from build123d import *

# Parameters (mm, degrees)
F0_R     = 4.05
F1_DEPTH = 50
F2_R     = 10.963605
F2_R_2   = 4.05
F3_DEPTH = 100


with BuildPart() as f1:
    # F0 (on Top) → F1 (new body)
    with BuildSketch(Plane.XY):
        with BuildLine():
            Line((14.85866, -53.070427), (16.429462, -41.893589))
            ThreePointArc((16.429462, -41.893589), (9.356026, -44.016642), (2.030598, -44.954162))
            Line((2.030598, -44.954162), (8.011626, -54.525809))
            Line((8.011626, -54.525809), (11.435143, -53.798118))
            Line((11.435143, -53.798118), (14.85866, -53.070427))
        make_face()
        with BuildLine():
            Line((-8.011626, -54.525809), (-2.030598, -44.954162))
            ThreePointArc((-2.030598, -44.954162), (-9.356026, -44.016642), (-16.429462, -41.893589))
            Line((-16.429462, -41.893589), (-14.85866, -53.070427))
            Line((-14.85866, -53.070427), (-11.435143, -53.798118))
            Line((-11.435143, -53.798118), (-8.011626, -54.525809))
        make_face()
        with BuildLine():
            Line((-29.496629, -46.553183), (-20.139548, -40.241752))
            ThreePointArc((-20.139548, -40.241752), (-26.450336, -36.405765), (-32.048718, -31.589234))
            Line((-32.048718, -31.589234), (-35.159748, -42.438686))
            Line((-35.159748, -42.438686), (-32.328189, -44.495935))
            Line((-32.328189, -44.495935), (-29.496629, -46.553183))
        make_face()
        with BuildLine():
            Line((-45.881397, -30.531089), (-34.766188, -28.571178))
            ThreePointArc((-34.766188, -28.571178), (-38.971143, -22.5), (-42.126459, -15.822813))
            Line((-42.126459, -15.822813), (-49.381397, -24.468911))
            Line((-49.381397, -24.468911), (-47.631397, -27.5))
            Line((-47.631397, -27.5), (-45.881397, -30.531089))
        make_face()
        with BuildLine():
            Line((-54.332855, -9.229892), (-43.381438, -11.960387))
            ThreePointArc((-43.381438, -11.960387), (-44.753485, -4.703781), (-44.920154, 2.679516))
            Line((-44.920154, 2.679516), (-55.064554, -2.268239))
            Line((-55.064554, -2.268239), (-54.698704, -5.749065))
            Line((-54.698704, -5.749065), (-54.332855, -9.229892))
        make_face()
        with BuildLine():
            ThreePointArc((-37.916147, 24.23563), (-33.441517, 30.110877), (-28.066181, 35.175126))
            Line((-28.066181, 35.175126), (-38.531008, 39.40319))
            Line((-38.531008, 39.40319), (-40.872965, 36.802183))
            Line((-40.872965, 36.802183), (-43.214923, 34.201176))
            Line((-43.214923, 34.201176), (-37.916147, 24.23563))
        make_face()
        with BuildLine():
            ThreePointArc((-44.495643, 6.718463), (-42.797543, 13.905765), (-39.946745, 20.718532))
            Line((-39.946745, 20.718532), (-51.226549, 20.324632))
            Line((-51.226549, 20.324632), (-52.308108, 16.995935))
            Line((-52.308108, 16.995935), (-53.389668, 13.667237))
            Line((-53.389668, 13.667237), (-44.495643, 6.718463))
        make_face()
        with BuildLine():
            ThreePointArc((-24.780606, 37.562236), (-18.303149, 41.109546), (-11.33272, 43.549621))
            Line((-11.33272, 43.549621), (-19.173106, 51.668578))
            Line((-19.173106, 51.668578), (-22.370515, 50.245))
            Line((-22.370515, 50.245), (-25.567924, 48.821422))
            Line((-25.567924, 48.821422), (-24.780606, 37.562236))
        make_face()
        with BuildLine():
            ThreePointArc((-7.360272, 44.393991), (0, 45), (7.360272, 44.393991))
            Line((7.360272, 44.393991), (3.5, 55))
            Line((3.5, 55), (0, 55))
            Line((0, 55), (-3.5, 55))
            Line((-3.5, 55), (-7.360272, 44.393991))
        make_face()
        with BuildLine():
            ThreePointArc((11.33272, 43.549621), (18.303149, 41.109546), (24.780606, 37.562236))
            Line((24.780606, 37.562236), (25.567924, 48.821422))
            Line((25.567924, 48.821422), (22.370515, 50.245))
            Line((22.370515, 50.245), (19.173106, 51.668578))
            Line((19.173106, 51.668578), (11.33272, 43.549621))
        make_face()
        with BuildLine():
            ThreePointArc((28.066181, 35.175126), (33.441517, 30.110877), (37.916147, 24.23563))
            Line((37.916147, 24.23563), (43.214923, 34.201176))
            Line((43.214923, 34.201176), (40.872965, 36.802183))
            Line((40.872965, 36.802183), (38.531008, 39.40319))
            Line((38.531008, 39.40319), (28.066181, 35.175126))
        make_face()
        with BuildLine():
            ThreePointArc((39.946745, 20.718532), (42.797543, 13.905765), (44.495643, 6.718463))
            Line((44.495643, 6.718463), (53.389668, 13.667237))
            Line((53.389668, 13.667237), (52.308108, 16.995935))
            Line((52.308108, 16.995935), (51.226549, 20.324632))
            Line((51.226549, 20.324632), (39.946745, 20.718532))
        make_face()
        with BuildLine():
            Line((49.381397, -24.468911), (42.126459, -15.822813))
            ThreePointArc((42.126459, -15.822813), (38.971143, -22.5), (34.766188, -28.571178))
            Line((34.766188, -28.571178), (45.881397, -30.531089))
            Line((45.881397, -30.531089), (47.631397, -27.5))
            Line((47.631397, -27.5), (49.381397, -24.468911))
        make_face()
        with BuildLine():
            ThreePointArc((43.381438, -11.960387), (44.593524, -6.034704), (45, 0))
            ThreePointArc((45, 0), (44.980034, 1.340353), (44.920154, 2.679516))
            ThreePointArc((44.920154, 2.679516), (44.753485, 4.703781), (44.495643, 6.718463))
            ThreePointArc((44.495643, 6.718463), (42.797543, 13.905765), (39.946745, 20.718532))
            ThreePointArc((39.946745, 20.718532), (38.971143, 22.5), (37.916147, 24.23563))
            ThreePointArc((37.916147, 24.23563), (33.441517, 30.110877), (28.066181, 35.175126))
            ThreePointArc((28.066181, 35.175126), (26.450336, 36.405765), (24.780606, 37.562236))
            ThreePointArc((24.780606, 37.562236), (18.303149, 41.109546), (11.33272, 43.549621))
            ThreePointArc((11.33272, 43.549621), (9.356026, 44.016642), (7.360272, 44.393991))
            ThreePointArc((7.360272, 44.393991), (0, 45), (-7.360272, 44.393991))
            ThreePointArc((-7.360272, 44.393991), (-9.356026, 44.016642), (-11.33272, 43.549621))
            ThreePointArc((-11.33272, 43.549621), (-18.303149, 41.109546), (-24.780606, 37.562236))
            ThreePointArc((-24.780606, 37.562236), (-26.450336, 36.405765), (-28.066181, 35.175126))
            ThreePointArc((-28.066181, 35.175126), (-33.441517, 30.110877), (-37.916147, 24.23563))
            ThreePointArc((-37.916147, 24.23563), (-38.971143, 22.5), (-39.946745, 20.718532))
            ThreePointArc((-39.946745, 20.718532), (-42.797543, 13.905765), (-44.495643, 6.718463))
            ThreePointArc((-44.495643, 6.718463), (-44.753485, 4.703781), (-44.920154, 2.679516))
            ThreePointArc((-44.920154, 2.679516), (-44.753485, -4.703781), (-43.381438, -11.960387))
            ThreePointArc((-43.381438, -11.960387), (-42.797543, -13.905765), (-42.126459, -15.822813))
            ThreePointArc((-42.126459, -15.822813), (-38.971143, -22.5), (-34.766188, -28.571178))
            ThreePointArc((-34.766188, -28.571178), (-33.441517, -30.110877), (-32.048718, -31.589234))
            ThreePointArc((-32.048718, -31.589234), (-26.450336, -36.405765), (-20.139548, -40.241752))
            ThreePointArc((-20.139548, -40.241752), (-18.303149, -41.109546), (-16.429462, -41.893589))
            ThreePointArc((-16.429462, -41.893589), (-9.356026, -44.016642), (-2.030598, -44.954162))
            ThreePointArc((-2.030598, -44.954162), (0, -45), (2.030598, -44.954162))
            ThreePointArc((2.030598, -44.954162), (9.356026, -44.016642), (16.429462, -41.893589))
            ThreePointArc((16.429462, -41.893589), (18.303149, -41.109546), (20.139548, -40.241752))
            ThreePointArc((20.139548, -40.241752), (26.450336, -36.405765), (32.048718, -31.589234))
            ThreePointArc((32.048718, -31.589234), (33.441517, -30.110877), (34.766188, -28.571178))
            ThreePointArc((34.766188, -28.571178), (38.971143, -22.5), (42.126459, -15.822813))
            ThreePointArc((42.126459, -15.822813), (42.797543, -13.905765), (43.381438, -11.960387))
        make_face()
        Circle(F0_R, mode=Mode.SUBTRACT)
        with BuildLine():
            Line((35.159748, -42.438686), (32.048718, -31.589234))
            ThreePointArc((32.048718, -31.589234), (26.450336, -36.405765), (20.139548, -40.241752))
            Line((20.139548, -40.241752), (29.496629, -46.553183))
            Line((29.496629, -46.553183), (32.328189, -44.495935))
            Line((32.328189, -44.495935), (35.159748, -42.438686))
        make_face()
        with BuildLine():
            ThreePointArc((44.920154, 2.679516), (44.980034, 1.340353), (45, 0))
            ThreePointArc((45, 0), (44.593524, -6.034704), (43.381438, -11.960387))
            Line((43.381438, -11.960387), (54.332855, -9.229892))
            Line((54.332855, -9.229892), (54.698704, -5.749065))
            Line((54.698704, -5.749065), (55.064554, -2.268239))
            Line((55.064554, -2.268239), (44.920154, 2.679516))
        make_face()
        Circle(F0_R)
    extrude(amount=F1_DEPTH)

    # F2 (on face) → F3 (cut)
    with BuildSketch(Plane.XY.offset(50)):
        with Locations((0, 25.067315)):
            Circle(F2_R)
        with Locations((-25.067315, 0)):
            Circle(F2_R)
        with Locations((25.067315, 0)):
            Circle(F2_R)
        Circle(F2_R_2)
        with Locations((0, -25.067315)):
            Circle(F2_R)
    extrude(amount=-F3_DEPTH, mode=Mode.SUBTRACT)


solid = f1.part
Source: CAD feature listing. Evaluate the final solid. Frame: model axes, mm. A direction names the side the tool comes from. Coordinates: 2 decimals unless noted, no trailing zeros. Order: outer loops, then holes, each group sorted by start corner. A loop starts at its lowest first (then second) coordinate and runs counter-clockwise, first axis right, second up. Notation, with made-up numbers: M -37,71 L 16,71 A28 cw 16,96 Z; hole C -38,40.5 d10. An arc over 180 degrees is marked long. Write each question's results on one line, items separated by ' | '. Start each with the question number.
1. Section A-A, the plane x = 0. Return the cut outline in (y, z), then the cut area to 3 significant figures.
2. Pin query (flat end, axial travel): pin 1 (2 mm diameter, centred on y = -17.5, z = 37, fed in from -X); pin 2 (3 mm diameter, centred on y = 43, z = 10, fed in from +X); pin 3 (10 mm diameter, centred on y = -33.5, z = 23, fed in from +X); pin 4 (1.5 mm diameter, centred on x = 43.5, y = 9, fed in from -Z). Return the tip coordinate at first contact, or that it passes through.
3. Draft query along Y for faces 4 (the face through (15.31, 47.67, 24.65)), 5 (the face through (47.61, -27.54, 24.65)), 6 (the face through (33.422, -30.132, 24.65)). Return one class per face: +Y half, -Y half, draft (parallel to the pull), parting line (faces both ways), or undercut.
4. Section C-C, the plane z = 44.5. State how many separate pieces and enclosed holes the cut face has, then the cut area to 3 significant figures.
5. Reachability of faces 1 (the face through (-26.43, 36.42, 24.65)), 2 (the face through (-15.655, -47.404, 24.65)), 3 (the face through (44.756, 4.675, 24.65)) from +Z, -Z, +X, -X, +Y, -Y: full face, straight path, thin tool, end or side. Return the list, or none.
6. Section B-B, the plane y = 0. Return the cut outline in (x, z).
7. Material intervals for L1, parallel to X at y = 0.5, z = 8.5; L2, parallel to Y at x = -0.5, z = 35; L3, parallel to X at y = 3, z = 43, sorted ascending.
Solution:
1) outline: M -45,0 L -36.03,0 L -36.03,50 L -45,50 Z; M -14.1,0 L -4.05,0 L -4.05,50 L -14.1,50 Z; M 4.05,0 L 14.1,0 L 14.1,50 L 4.05,50 Z; M 36.03,0 L 55,0 L 55,50 L 36.03,50 Z | area: 2,400 mm²
2) pin 1: x = -44.37 | pin 2: x = 25.27 | pin 3: x = 47.05 | pin 4: z = 0
3) face 4: +Y half | face 5: -Y half | face 6: undercut
4) separate pieces: 1 | enclosed holes: 5 | area: 6,440 mm²
5) face 1: +Z, -Z | face 2: +Z, -Z, -Y | face 3: +Z, -Z, +X
6) outline: M -50.41,0 L -36.03,0 L -36.03,50 L -50.41,50 Z; M -14.1,0 L -4.05,0 L -4.05,50 L -14.1,50 Z; M 4.05,0 L 14.1,0 L 14.1,50 L 4.05,50 Z; M 36.03,0 L 50.41,0 L 50.41,50 L 36.03,50 Z
7) L1: -49.39 to -36.02, -14.12 to -4.02, 4.02 to 14.12, 36.02 to 49.39 | L2: -45 to -36.02, -14.12 to -4.02, 4.02 to 14.12, 36.02 to 55 | L3: -44.9 to -35.61, -14.52 to -2.72, 2.72 to 14.52, 35.61 to 44.9
